The listing builds one solid part. Answer for the finished solid, in the listing's coordinates (mm). Face numbers are marked on the shaded views. A direction names the side the tool comes from. Round coordinates to 2 decimals unless told otherwise and drop trailing zeros. Write each loop counter-clockwise with the first axis right and the second up, starting at its lowest first coordinate (ties: lowest second). Pieces come first, ordered by that corner, then holes.
Item 1: Find the intervals of material crossed by probe 1 along Z at (x, y) = (53, 27) (3 decimals); probe 2 along Y at (x, z) = (79.5, -23.5); probe 3 along X at (y, z) = (-37.5, -48), in increasing order.
Item 2: For a pull along Y with two mould halves and no side action, classify the marked faces 3, 4, 5 and 6 as +Y half, -Y half, draft (parallel to the pull), parting line (faces both ways), or undercut.
Item 3: A tool of negligible diameter and unlimited length cuts with its end or side. For the marked faces 1 and 2, from which of +Z, -Z, +X, -X, +Y, -Y can it reach the whole face along a straight path? Write none if from no direction.
Item 4: Find section C-C on y = 54.5. Give the vertices of the cut face in (x, z) (3 decimals).
Item 5: Find section A-A on y = 13. Give the vertices of the cut face in (x, z) (3 decimals), then the cut area to 3 significant figures.
Item 6: Each of these flat-tipped pins is pushed along its axis until it touches: pin 1 (4 mm diameter, centred on x = 105.5, y = -32.5, fed in from +Z); pin 2 (1.5 mm diameter, centred on x = 64, z = 5.5, fed in from -Y); pin 3 (1.5 mm diameter, centred on x = 85.5, y = -26.5, fed in from +Z). Where does it stop, or does it pass through?
Item 7: Find section D-D on z = 16. Give the vertices of the cut face in (x, y).
Item 8: Find section B-B on x = 118. Give the vertices of the cut face in (y, z) (3 decimals).
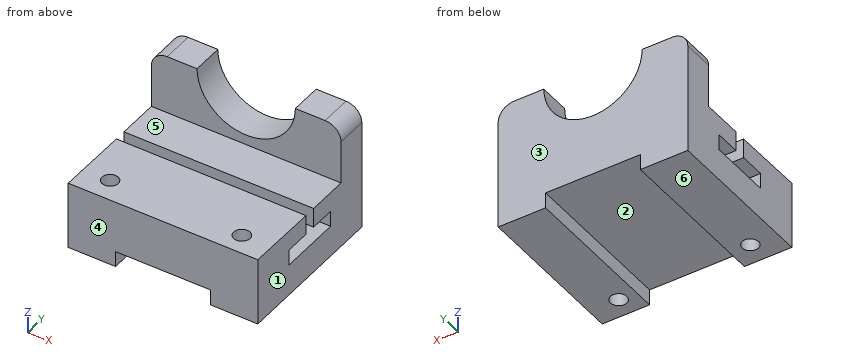
```python
from build123d import *

# Parameters (mm, degrees)
F1_DEPTH = 152.4
F2_W     = 76.2
F2_H     = 12.7
F3_DEPTH = 127.001
F4_R     = 39.507453211
F5_DEPTH = 25.4
F6_R     = 12.7
F7_R     = 6.6080051974
F7_R_2   = 6.5366056143
F8_DEPTH = 54.6147514972


with BuildPart() as f1:
    # F0 (on Right) → F1 (new body)
    with BuildSketch(Plane.YZ):
        Polygon((68.1480239093, 47.625), (42.7480239093, 47.625), (42.7480239093, 0), (9.2960478187, 0), (9.2960478187, -15.875), (30.0480239093, -15.875), (30.0480239093, -28.575), (-20.7519760907, -28.575), (-20.7519760907, -15.875), (0, -15.875), (0, 0), (-58.8519760907, 0.6420009357), (-58.8519760907, -53.975), (68.1480239093, -53.975), align=None)
    extrude(amount=F1_DEPTH)

    # F2 (on face) → F3 (cut, through all)
    with BuildSketch(Plane.XZ.offset(58.8519760907)):
        with Locations((76.2, -47.625)):
            Rectangle(F2_W, F2_H)
    extrude(amount=-F3_DEPTH, mode=Mode.SUBTRACT)

    # F4 (on face) → F5 (cut)
    with BuildSketch(Plane.XZ.offset(-42.7480239093)):
        with Locations((76.2, 47.625)):
            Circle(F4_R)
        with BuildLine():
            ThreePointArc((36.692546789, 47.625), (76.2, 8.117546789), (115.707453211, 47.625))
            Line((115.707453211, 47.625), (36.692546789, 47.625))
        make_face()
    extrude(amount=-F5_DEPTH, mode=Mode.SUBTRACT)

    # F6
    f6_edges = [f1.edges().sort_by_distance(p)[0] for p in [
        (152.4, 55.448024, 47.625),
        (0, 55.448024, 47.625),
    ]]
    fillet(f6_edges, radius=F6_R)

    # F7 (on face) → F8 (cut, through all)
    with BuildSketch(Plane(origin=(0, 0, 0), x_dir=(1, 0, 0), z_dir=(0, 0.0109080915, 0.999940505))):
        with Locations((128.5557597876, -42.1188808978)):
            Circle(F7_R)
        with Locations((21.6534994543, -40.5630394816)):
            Circle(F7_R_2)
    extrude(amount=-F8_DEPTH, mode=Mode.SUBTRACT)


solid = f1.part
```
Check values:
1. probe 1: z = -41.275 to -28.575, -15.875 to 0
1. probe 2: y = -58.85 to -20.75, 30.05 to 68.15
1. probe 3: x = 0 to 16.19, 27.12 to 38.1, 114.3 to 124.41, 132.7 to 152.4
2. face 3: +Y half
2. face 4: -Y half
2. face 5: undercut
2. face 6: draft
3. face 1: +Z, -Z, +X, +Y, -Y
3. face 2: -Z, +Y, -Y
4. outline: (0, -53.975) - (38.1, -53.975) - (38.1, -41.275) - (114.3, -41.275) - (114.3, -53.975) - (152.4, -53.975) - (152.4, 34.925) arc R12.7 ccw to (139.7, 47.625) - (115.707, 47.625) arc R39.507 cw to (36.693, 47.625) - (12.7, 47.625) arc R12.7 ccw to (0, 34.925) - close
5. outline: (0, -53.975) - (38.1, -53.975) - (38.1, -41.275) - (114.3, -41.275) - (114.3, -53.975) - (152.4, -53.975) - (152.4, -28.575) - (0, -28.575) - close; (0, -15.875) - (152.4, -15.875) - (152.4, 0) - (0, 0) - close
5. area: 5,320 mm2
6. pin 1: stops at z = 0.38
6. pin 2: stops at y = 42.75
6. pin 3: stops at z = 0.3
7. outline: (0, 42.75) - (52.52, 42.75) - (52.52, 68.15) - (0, 68.15) - close; (99.88, 42.75) - (152.4, 42.75) - (152.4, 68.15) - (99.88, 68.15) - close
8. outline: (-58.852, -53.975) - (68.148, -53.975) - (68.148, 47.625) - (42.748, 47.625) - (42.748, 0) - (9.296, 0) - (9.296, -15.875) - (30.048, -15.875) - (30.048, -28.575) - (-20.752, -28.575) - (-20.752, -15.875) - (0, -15.875) - (0, 0) - (-58.852, 0.642) - close
